```python
from build123d import *

# Parameters (mm, degrees)
F1_DEPTH = 7.79
F2_DEPTH = 3.46
F3_R     = 2.875
F4_DEPTH = 5.5
F5_R     = 1.8
F7_R     = 2.75
F8_DEPTH = 7.35


with BuildPart() as f1:
    # F0 (on Top) → F1 (new body, symmetric)
    with BuildSketch(Plane.XY):
        Polygon((-2.75, 101.27), (2.75, 101.27), (11.46, 101.27), (11.46, 139.82), (-11.46, 139.82), (-11.46, 101.27), align=None)
    extrude(amount=F1_DEPTH, both=True)



with BuildPart() as f2:
    # F0 (on Top) → F2 (new body, symmetric)
    with BuildSketch(Plane.XY):
        Polygon((-4.94, -10.92), (4.94, -10.92), (4.94, 10.92), (2.875, 10.92), (-2.875, 10.92), (-4.94, 10.92), align=None)
    extrude(amount=F2_DEPTH, both=True)

    # F3 (on face) → F4 (join, through all)
    with BuildSketch(Plane(origin=(0, 10.92, 0), x_dir=(-1, 0, 0), z_dir=(0, 1, 0))):
        Circle(F3_R)
    extrude(amount=F4_DEPTH)

    # F6: sweep along a path in F0
    with BuildLine(Plane.XY) as f6_path:
        Line((1.8, 16.42), (1.8, 93.92))
    # F5 (on face) → F6 (sweep)
    with BuildSketch(Plane(origin=(0, 16.42, 0), x_dir=(-1, 0, 0), z_dir=(0, 1, 0))):
        Circle(F5_R)
    sweep(path=f6_path.line)


with BuildPart() as f1_1:
    add(f1.part)

    add(f2.part)  # F8 merges F2
    # F7 (on face) → F8 (join, through all)
    with BuildSketch(Plane.XZ.offset(-101.27)):
        Circle(F7_R)
    extrude(amount=F8_DEPTH)


solid = f1_1.part
```
Source: CAD feature listing. Evaluate the final solid. Frame: model axes, mm. A direction names the side the tool comes from. Coordinates: 2 decimals unless noted, no trailing zeros. Write each loop counter-clockwise with the first axis right and the second up, starting at its lowest first coordinate (ties: lowest second). Pieces come first, ordered by that corner, then holes. Notation, with made-up numbers: (74.5, 80) -> (109.5, 80) arc R21 cw to (109.5, 116) -> close; hole circle Ø1 at (73, 37.5). An arc over 180 degrees is marked (long way). Return JSON: item names as keys, results as strings. Group by question number.
1) Section query A-A, the plane z = 0. Return loops of the section in (x, y) (3 decimals), plus the area to 3 significant figures.
2) Set-up query: faces 4 (the face through (-2, 16.42, 0)), 5 (the face through (-4.94, 0, 0)), 6 (the face through (0, 0, 3.46)). Return all of +Z, -Z, +X, -X, +Y, -Y with unobstructed straight access to the full face (end or side cutting, diameter ignored); none if empty.
3) Section query B-B, the plane x = 0. Return loops of the section in (y, z) (3 decimals), plus the area to 3 significant figures.
4) Ray query, line 1 along Y through (x, z) = (2.5, 1.75); line 2 along Y through (x, z) = (1, -2); line 3 along Y through (x, z) = (-8, 7). Return the intervals inside material, ascending.
5) Section query C-C, the plane y = 44.5. Return loops of the section in (x, z), plus the area to 3 significant figures.
6) Contact query for flat-ended pins moving along their axis: P1, Ø3, axis at x = 1.5, y = 5, coming from the -Z side; P2, Ø5.5, axis at y = -2, z = 1.5, coming from the +X side; P3, Ø3.5, axis at y = -4.5, z = -1, coming from the -X side. Output: stop coordinate, or through.
7) Mould query, pull axis Y, two halves, no side actions, for faces 1 (the face through (0, 139.82, 0)), 2 (the face through (0.37, 13.63, 2.85)), 3 (the face through (11.46, 120, 0)). Classes: +Y half, -Y half, draft (parallel to the pull), parting line (faces both ways), or undercut.
8) Section query D-D, the plane x = 8.75. Return loops of the section in (y, z).
From the geometry:
{
 "1": {"outline": "(-11.46, 101.27) -> (-2.75, 101.27) -> (-2.75, 93.92) -> (-1.8, 93.92) -> (-1.8, 16.42) -> (-2.875, 16.42) -> (-2.875, 10.92) -> (-4.94, 10.92) -> (-4.94, -10.92) -> (4.94, -10.92) -> (4.94, 10.92) -> (2.875, 10.92) -> (2.875, 16.42) -> (1.8, 16.42) -> (1.8, 93.92) -> (2.75, 93.92) -> (2.75, 101.27) -> (11.46, 101.27) -> (11.46, 139.82) -> (-11.46, 139.82) -> close", "area": "1,450 mm²"},
 "2": {"face 4": "none", "face 5": "+Z, -Z, -X, -Y", "face 6": "+Z, +X, -X, -Y"},
 "3": {"outline": "(-10.92, -3.46) -> (10.92, -3.46) -> (10.92, -2.875) -> (16.42, -2.875) -> (16.42, -1.8) -> (93.92, -1.8) -> (93.92, -2.75) -> (101.27, -2.75) -> (101.27, -7.79) -> (139.82, -7.79) -> (139.82, 7.79) -> (101.27, 7.79) -> (101.27, 2.75) -> (93.92, 2.75) -> (93.92, 1.8) -> (16.42, 1.8) -> (16.42, 2.875) -> (10.92, 2.875) -> (10.92, 3.46) -> (-10.92, 3.46) -> close", "area": "1,100 mm²"},
 "4": {"line 1": "-10.92 to 10.92, 101.27 to 139.82", "line 2": "-10.92 to 16.42, 93.92 to 139.82", "line 3": "101.27 to 139.82"},
 "5": {"outline": "circle Ø3.6 at (0, 0)", "area": "10.2 mm²"},
 "6": {"P1": "z = -3.46", "P2": "x = 4.94", "P3": "x = -4.94"},
 "7": {"face 1": "+Y half", "face 2": "undercut", "face 3": "draft"},
 "8": {"outline": "(101.27, -7.79) -> (139.82, -7.79) -> (139.82, 7.79) -> (101.27, 7.79) -> close"}
}
